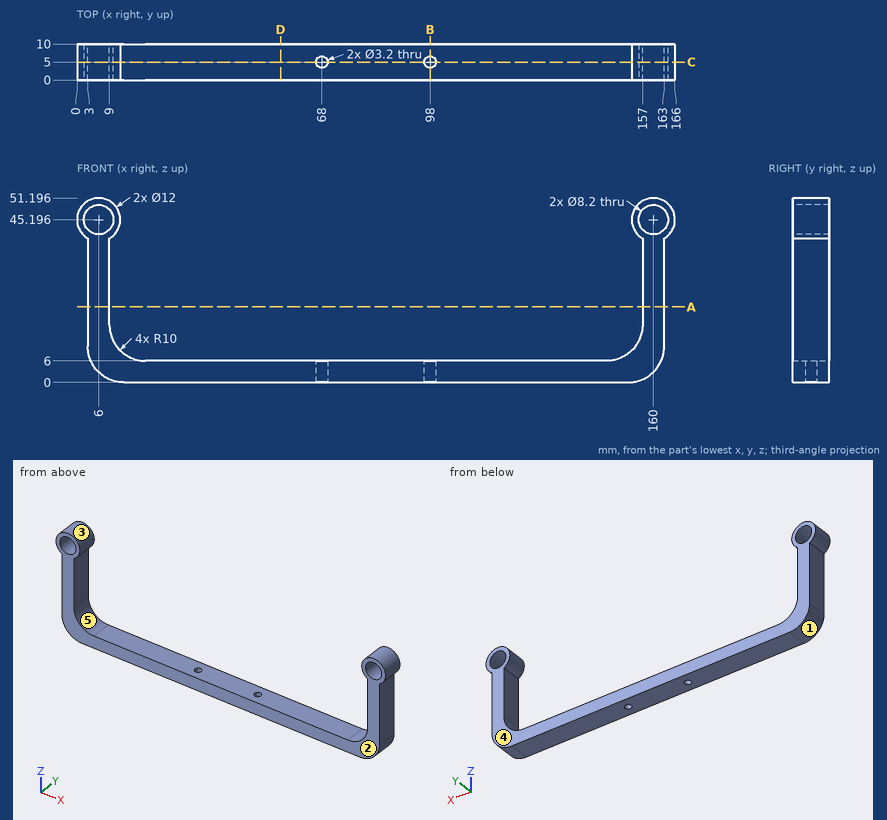
Geometry: see drawing. Coordinates: mm, zero at the bounding-box minimum. A direction names the side the tool comes from. Coordinates: 2 decimals unless noted, no trailing zeros. Loops run counter-clockwise (first coordinate to the right, second up) from the corner with the lowest first, then second, coordinate; pieces in that order, holes last.
(1) Set-up query: the marked faces 4 and 5. Return all of +Z, -Z, +X, -X, +Y, -Y with unobstructed straight access to the full face (end or side cutting, diameter ignored); none if empty.
(2) Section A-A on z = 21. Return the cut outline in (x, y).
(3) Section C-C on y = 5. Return the cut outline in (x, z), then the cut area to 3 significant figures.
(4) Material intervals for probe 1 along X at (y, z) = (4, 16); probe 2 along Y at (x, z) = (68, 4); probe 3 along X at (y, z) = (2, 15), sorted ascending.
(5) Section D-D on x = 56.5. Return the cut outline in (y, z).
(6) Pull-direction query (X, two-part tool) for the marked faces 1, 2 and 3; classes: released by +X, released by -X, zero draft, split by the parting line, or undercut.
(7) Section B-B on x = 98. Return the cut outline in (y, z).
(8) First-contact query: pin 1 Ø2 at (y, z) = (2.5, 24) entering from -X; pin 2 Ø5 at (y, z) = (5, 17.5) entering from +X; pin 3 Ø3 at (x, y) = (75.5, 5) entering from +Z. Flat tips, straight axial feed; report the tip coordinate or a pass-through.
Data:
1. face 4: +Z, -Z, +X, -X, +Y
1. face 5: +Y, -Y
2. outline: (3, 0) - (9, 0) - (9, 10) - (3, 10) - close; (157, 0) - (163, 0) - (163, 10) - (157, 10) - close
3. outline: (3, 10) arc R10 ccw to (13, 0) - (66.4, 0) - (66.4, 6) - (19, 6) arc R10 cw to (9, 16) - (9, 40) arc R6 ccw (long way) to (3, 40) - close; (69.6, 0) - (96.4, 0) - (96.4, 6) - (69.6, 6) - close; (99.6, 0) - (153, 0) arc R10 ccw to (163, 10) - (163, 40) arc R6 ccw (long way) to (157, 40) - (157, 16) arc R10 cw to (147, 6) - (99.6, 6) - close; hole circle Ø8.2 at (6, 45.2); hole circle Ø8.2 at (160, 45.2)
3. area: 1,440 mm2
4. probe 1: x = 3 to 9, 157 to 163
4. probe 2: y = 0 to 3.4, 6.6 to 10
4. probe 3: x = 3 to 9.05, 156.95 to 163
5. outline: (0, 0) - (10, 0) - (10, 6) - (0, 6) - close
6. face 1: released by -X
6. face 2: zero draft
6. face 3: undercut
7. outline: (0, 0) - (3.4, 0) - (3.4, 6) - (0, 6) - close; (6.6, 0) - (10, 0) - (10, 6) - (6.6, 6) - close
8. pin 1: stops at x = 3
8. pin 2: stops at x = 163
8. pin 3: stops at z = 6
